from build123d import *

# Parameters (mm, degrees)
F0_W     = 75.2
F0_H     = 53.2
F1_DEPTH = 4
F2_R     = 0.75
F3_DEPTH = 2
F5_DEPTH = 25


with BuildPart() as f1:
    # F0 (on Top) → F1 (new body)
    with BuildSketch(Plane.XY):
        with Locations((37.6, -26.6)):
            Rectangle(F0_W, F0_H)
    extrude(amount=F1_DEPTH)

    # F2 (on face) → F3 (join)
    with BuildSketch(Plane.XY.offset(4)):
        with Locations((10.5, -10)):
            Circle(F2_R)
        with Locations((63.7, -49.2)):
            Circle(F2_R)
        with Locations((64.7, -10.5)):
            Circle(F2_R)
    extrude(amount=F3_DEPTH)

    # F4 (on face) → F5 (cut)
    with BuildSketch(Plane.XY.offset(4)):
        Polygon((20, -20), (10, -20), (10, -43.2), (55.2, -43.2), (55.2, -38.2), (65.2, -38.2), (65.2, -20), (55.2, -20), (55.2, -10), (20, -10), align=None)
    extrude(amount=-F5_DEPTH, mode=Mode.SUBTRACT)


solid = f1.part
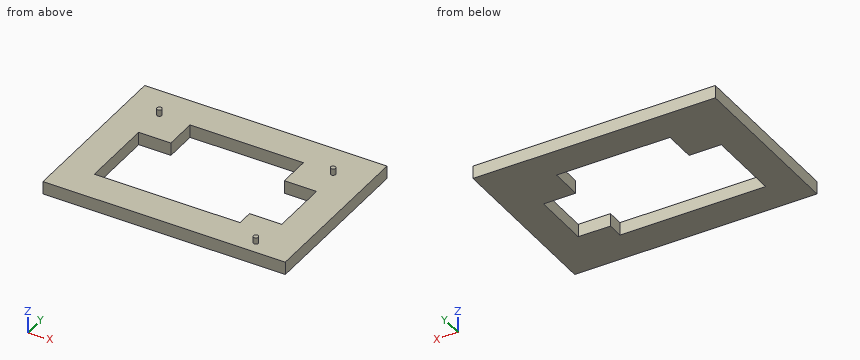
Work out the finished part from the listing and answer in its coordinate system (mm). Round coordinates to 2 decimals unless told otherwise and drop trailing zeros. Order: outer loops, then holes, each group sorted by start corner. A loop starts at its lowest first (then second) coordinate and runs counter-clockwise, first axis right, second up. Notation, with made-up numbers: M 74.5,-40 L 107.5,-40 A17 ccw 107.5,-25 Z; hole C 21,86 d1. An arc over 180 degrees is marked long. One line per item, written item: value.
Q1. Find section C-C on x = 42. Write down the section's boundary in (y, z), then the cut area to 3 significant figures.
Derived:
outline: M -53.2,0 L -43.2,0 L -43.2,4 L -53.2,4 Z; M -10,0 L 0,0 L 0,4 L -10,4 Z
area: 80.0 mm²
Q2. Find section A-A on y = -19. Write down the section's boundary in (x, z), then the cut area to 3 significant figures.
Derived:
outline: M 0,0 L 20,0 L 20,4 L 0,4 Z; M 55.2,0 L 75.2,0 L 75.2,4 L 55.2,4 Z
area: 160 mm²
Q3. Find section D-D on y = -49.2. Write down the section's boundary in (x, z), then the cut area to 3 significant figures.
Derived:
outline: M 0,0 L 75.2,0 L 75.2,4 L 64.45,4 L 64.45,6 L 62.95,6 L 62.95,4 L 0,4 Z
area: 304 mm²
Q4. Find section B-B on z = 2. Write down the section's boundary in (x, y), then the cut area to 3 significant figures.
Derived:
outline: M 0,-53.2 L 75.2,-53.2 L 75.2,0 L 0,0 Z; hole M 10,-43.2 L 55.2,-43.2 L 55.2,-38.2 L 65.2,-38.2 L 65.2,-20 L 55.2,-20 L 55.2,-10 L 20,-10 L 20,-20 L 10,-20 Z
area: 2,420 mm²
Q5. Flat-ended cylindrical pins translate along their axes: pin 1 (2 mm diameter, centred on x = 57, y = -37.5, fed in from +Z); pin 2 (3 mm diameter, centred on x = 59.5, y = -22.5, fed in from -Z). Find the tip coordinate at first contact, or state that the pin passes through.
Derived:
pin 1: z = 4
pin 2: through
Q6. Straight lines are drawn through the part: line 1 (X direction, y = -24, z = 2.9); line 2 (X direction, y = -43, z = 2); line 3 (Y direction, x = 30.5, z = 2.6). For each, find the intervals that lie inside material, in ascending order.
Derived:
line 1: 0 to 10, 65.2 to 75.2
line 2: 0 to 10, 55.2 to 75.2
line 3: -53.2 to -43.2, -10 to 0
